Can you work these out from the drawing? Everything is in mm from the part's minimum corner. Round coordinates to 2 decimals unless told otherwise and drop trailing zeros. Order: outer loops, then holes, each group sorted by start corner. A loop starts at its lowest first (then second) coordinate and runs counter-clockwise, first axis right, second up. Notation, with made-up numbers: (-12, 81) -> (-6, 81) arc R33 ccw to (-6, 112) -> close; hole circle Ø11 at (83, -0.5). An arc over 180 degrees is marked (long way). One line per item, written item: value.
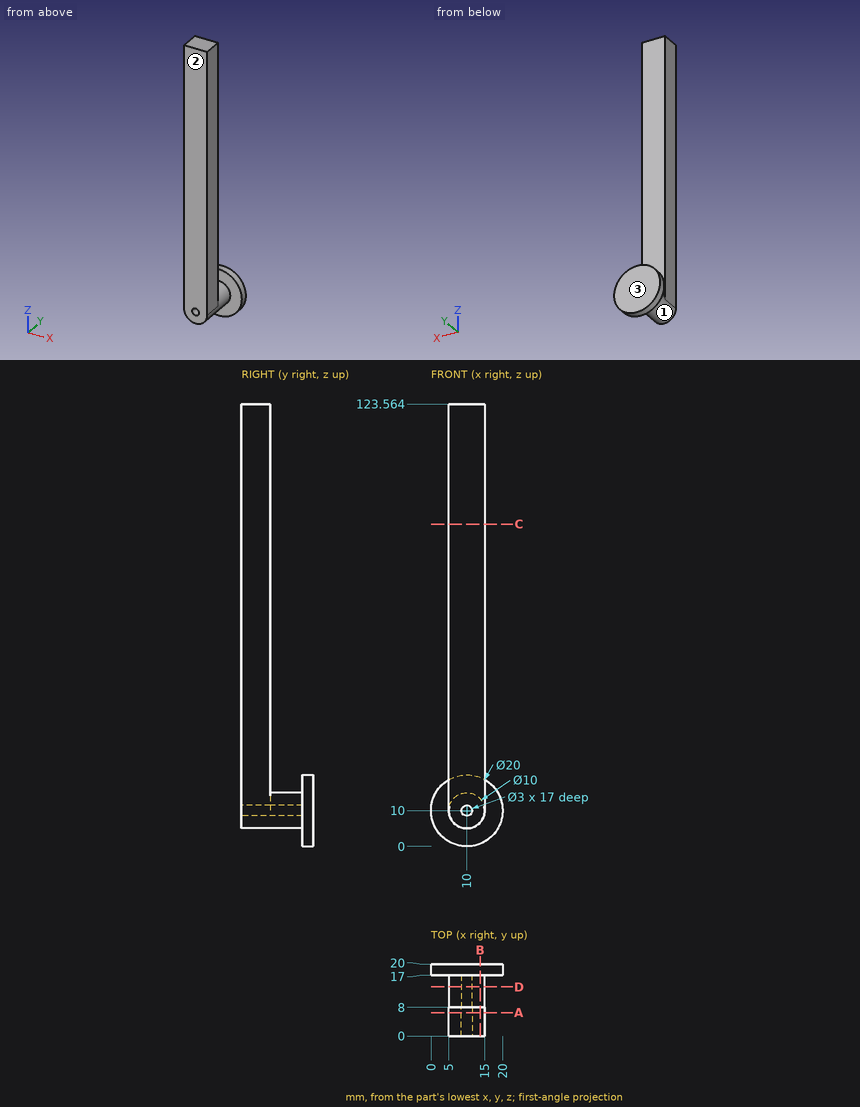
Q1. I want a section at D-D on y = 13.75. Write out the boundary of the cut face in (x, z), then the cut area to 3 significant figures.
Answers:
outline: circle Ø10 at (10, 10); hole circle Ø3 at (10, 10)
area: 71.5 mm2
Q2. For P1, Ø4, axis at y = 3.5, z = 50, coming from the +X side; P2, Ø2.5, axis at x = 10, z = 10, coming from the -Y side; P3, Ø3, axis at y = 7, z = 14, coming from the -X side, each with a flat end and sliding along its axis, tell me the tip position at first contact or that it passes through.
Answers:
P1: x = 15
P2: y = 17
P3: x = 5
Q3. I need wall thicknesses on line 1 along X through (y, z) = (5.5, 10); line 2 along Y through (x, z) = (8.25, 17). Which ranges of each line are inside material? Lowest first, please.
Answers:
line 1: 5 to 8.5, 11.5 to 15
line 2: 0 to 8, 17 to 20
Q4. If we mould it in two halves opening along Y, with no side actions, what happens to the marked faces 1, 2 and 3? For each: pulls with the +Y half, pulls with the -Y half, needs draft (parallel to the pull), parting line crosses it, or undercut.
Answers:
face 1: undercut
face 2: pulls with the -Y half
face 3: pulls with the +Y half
Q5. I want a section at B-B on x = 13.75. Write out the boundary of the cut face in (y, z).
Answers:
outline: (0, 6.69) -> (17, 6.69) -> (17, 0.73) -> (20, 0.73) -> (20, 19.27) -> (17, 19.27) -> (17, 13.31) -> (8, 13.31) -> (8, 123.56) -> (0, 123.56) -> close
Q6. I want a section at C-C on z = 90. Write out the boundary of the cut face in (x, y).
Answers:
outline: (5, 0) -> (15, 0) -> (15, 8) -> (5, 8) -> close
Q7. I want a section at A-A on y = 6.5. Write out the boundary of the cut face in (x, z), then the cut area to 3 significant figures.
Answers:
outline: (5, 10) arc R5 ccw to (15, 10) -> (15, 123.56) -> (5, 123.56) -> close; hole circle Ø3 at (10, 10)
area: 1,170 mm2
